Autodesk Inventor part; units mm, degrees
ref_plane "YZ Plane" through (0, 0, 0) normal (1, 0, 0) x (0, 1, 0)
ref_plane "XZ Plane" through (0, 0, 0) normal (0, 1, 0) x (-1, 0, 0)
ref_plane "XY Plane" through (0, 0, 0) normal (0, 0, 1) x (1, 0, 0)
sketch "Skizze1" plane through (0, 0, 0) normal (0, 0, 1) x (1, 0, 0)
  line L0 (0, 9.6853) -> (0, -8.6142)
  line L1 (-61.4142, 0) -> (18.4853, 0)
  arc A0 (3.5355, -3.5355) -> (-3.5355, 3.5355) centre (0, 0) ccw
  line L2 (-8.0711, -1) -> (-50, -1)
  line L3 (-50, -1) -> (-50, -6)
  line L4 (-50, -6) -> (1.0711, -6)
  line L5 (3.5355, -3.5355) -> (1.0711, -6)
  line L6 (-8.0711, -1) -> (-3.5355, 3.5355)
  dimension "d1" = 5
  dimension "d2" = 1
  dimension "d3" = 5
  dimension "d21" = 50
  dimension "d22" = 45
extrude "Extrusion1" add sketch "Skizze1" along normal blind 2
sketch "Skizze2" plane through (0, 0, 0) normal (0, 0, 1) x (1, 0, 0)
  point P0 (0, 0)
  point P1 (0, 0)
hole "Bohrung1" at (0, 0, 0) direction (0, 0, 1) diameter 2.9 end through all
sketch "Skizze5" plane through (-50, -6, 0) normal (-1, 0, 0) x (0, 0, 1)
  line L0 (0, 5) -> (0, 0)
  line L1 (0, 0) -> (2, 0)
  line L2 (2, 5) -> (2, 0)
  line L3 (0, 5) -> (2, 5)
  line L4 (0, 0) -> (2, 0)
  line L5 (0, 0) -> (-2, 2.3835)
  line L6 (-2, 2.3835) -> (-2, 3)
  line L7 (0, 5) -> (0, 0)
  line L8 (0, 0) -> (0, 5)
  line L9 (-2, 3) -> (-4.6, 3)
  line L10 (-4.6, 3) -> (-4.6, 5)
  line L11 (-4.6, 5) -> (0, 5)
  point P0 (0, 6)
  dimension "d23" = 40
  dimension "d28" = 3
  dimension "d29" = 2
  dimension "d30" = 4.6
extrude "Extrusion4" add sketch "Skizze5" against normal blind 5 contours L0 L5 L6 L9 L10 L11
fillet "Rundung1" radius 2 3 edges at (1.0711, -6, 1) (-8.0711, -1, 1) (-50, -6, 1)
sketch "Skizze8" plane through (0, 0, 0) normal (0, 0, -1) x (-1, 0, 0)
  circle A0 centre (0, 0) radius 5
  arc A1 (3.5355, 3.5355) -> (-3.5355, -3.5355) centre (0, 0) ccw
  circle A2 centre (0, 0) radius 1.45
  circle A3 centre (0, 0) radius 3
  dimension "d41" = 6
extrude "Extrusion7" add sketch "Skizze8" along normal blind 9.8 contours A3
sketch "Skizze6" plane through (0, 0, -9.8) normal (0, 0, -1) x (-1, 0, 0)
  circle A0 centre (0, 0) radius 1.5
  circle A1 centre (0, 0) radius 1.45
  circle A2 centre (0, 0) radius 1.45
  dimension "d32" = 3
extrude "Extrusion5" [suppressed]
sketch "Skizze7" plane through (0, 0, -12.2) normal (0, 0, -1) x (-1, 0, 0)
  line L0 (0.2, 2) -> (-0.2, 2)
  line L1 (-0.2, 2) -> (-0.2, -2)
  line L2 (-0.2, -2) -> (0.2, -2)
  line L3 (0.2, -2) -> (0.2, 2)
  line L4 (0.2, 2) -> (-0.2, -2) construction
  line L5 (-0.2, 2) -> (0.2, -2) construction
  point P0 (0, 0)
  dimension "d35" = 0.4
  dimension "d36" = 4
extrude "Extrusion6" [suppressed]
sketch "Skizze9" plane through (0, 0, 0) normal (0, 0, -1) x (-1, 0, 0)
  arc A0 (3.5355, 3.5355) -> (-3.5355, -3.5355) centre (0, 0) ccw
  circle A1 centre (0, 0) radius 5
  circle A2 centre (0, 0) radius 3
  point P0 (3.5355, 3.5355)
extrude "Extrusion8" add sketch "Skizze9" along normal blind 7
properties part number "Akkusperre"
Check sheet for the modelled part. Datum: model origin and axes. Units: mm. A direction names the side the tool comes from. Round coordinates to 2 decimals unless told otherwise and drop trailing zeros. Loops run counter-clockwise (first coordinate to the right, second up) from the corner with the lowest first, then second, coordinate; pieces in that order, holes last.
1. Sectioned sample at B-B on x = -2. Record the boundary of the cut face in (y, z).
2. Sectioned sample at A-A on z = -4. Record the boundary of the cut face in (x, y).
3. Sectioned sample at D-D on x = -18.5. Record the boundary of the cut face in (y, z).
4. Scan lines: probe 1 along X at (y, z) = (0, -5.25); probe 2 along Z at (x, y) = (-33.5, -3). Record each from-to range of solid material in increasing order.
5. Mould release check, pull along X, two halves, no side actions. Record for faces 1 (the flat face through (-5.54, 1.53, 0.99)), 2 (the flat face through (-48, -2, -4.6)), 3 (the cylindrical face through (0.896, 1.14, -3.817)): released by +X, released by -X, zero draft, split by the parting line, or undercut.
6. Gauge pin test, flat ends, axial feed: pin 1 Ø2 at (x, z) = (-38.5, 0) entering from +Y; pin 2 Ø6 at (y, z) = (2.5, -4.5) entering from -X; pin 3 Ø1 at (y, z) = (2, -6.5) entering from -X. Record the tip position at first contact, or that the pin passes through.
7. Set-up check for faces 4 (the flat face through (-47.54, -4.82, -0.99)), 5 (the flat face through (0.1, -3.3, -7)), 6 (the flat face through (-34, -1, 1)), 7 (the flat face through (-45, -2, -2)), 8 (the flat face through (2.61, -4.46, 0.99)): record each of +Z, -Z, +X, -X, +Y, -Y from which the full face is reachable in a straight line by a thin tool's end or side.
8. Sectioned sample at C-C on y = -2.5. Record the boundary of the cut face in (x, z).
Recorded:
1. outline: (-6, 0) - (-4.58, 0) - (-4.58, -7) - (-2.24, -7) - (-2.24, -9.8) - (2.24, -9.8) - (2.24, -7) - (4.58, -7) - (4.58, 2) - (-6, 2) - close
2. outline: (-50, -3) - (-45, -3) - (-45, -1) - (-50, -1) - close; circle Ø10 at (0, 0); hole circle Ø2.9 at (0, 0)
3. outline: (-6, 0) - (-1, 0) - (-1, 2) - (-6, 2) - close
4. probe 1: x = -5 to -1.45, 1.45 to 5
4. probe 2: z = 0 to 2
5. face 1: released by -X
5. face 2: zero draft
5. face 3: undercut
6. pin 1: stops at y = -1
6. pin 2: stops at x = -5
6. pin 3: stops at x = -4.77
7. face 4: -Z, -X, -Y
7. face 5: -Z
7. face 6: +Z, -Z, -X, +Y
7. face 7: -Z, +Y, -Y
7. face 8: +Z, -Z, +X, -Y
8. outline: (-50, -4.6) - (-45, -4.6) - (-45, 0) - (-4.33, 0) - (-4.33, -7) - (-1.66, -7) - (-1.66, -9.8) - (1.66, -9.8) - (1.66, -7) - (4.33, -7) - (4.33, 2) - (-50, 2) - close
